Autodesk Inventor part; units mm, degrees
ref_plane "Plano de trabalho1" through (-46, 6, -51.528) normal (0, -1, 0) x (1, 0, 0)
ref_plane "YZ Plane" through (0, 0, 0) normal (1, 0, 0) x (0, 1, 0)
ref_plane "XZ Plane" through (0, 0, 0) normal (0, 1, 0) x (-1, 0, 0)
ref_plane "Plano de trabalho1" through (-46, 6, -51.528) normal (0, -1, 0) x (1, 0, 0)
sketch "Esboço5" plane through (0, 0, 0) normal (0, 1, 0) x (-1, 0, 0)
  line L0 (51.75, 50.222) -> (51.75, -56.778)
  line L1 (38.75, -49.9946) -> (38.75, -21.778)
  line L2 (51.75, -21.778) -> (51.75, -56.778)
  line L3 (38.75, -21.778) -> (-37.25, -21.778)
  line L4 (-37.25, -21.778) -> (-37.25, -49.9946)
  line L5 (-37.25, -49.9946) -> (38.75, -49.9946)
  line L6 (51.75, 50.222) -> (-51.75, 50.222)
  line L7 (-51.75, 50.222) -> (-51.75, -56.778)
  line L8 (-51.75, -56.778) -> (51.75, -56.778)
  point P0 (0, 0)
  dimension "d24" = 76
  dimension "d28" = 51.75
  dimension "d30" = 103.5
extrude "Extrusão4" add sketch "Esboço5" against normal blind 3 from surface at 6
sketch "Esboço6" plane through (-51.75, 3, 50.222) normal (0, -1, 0) x (1, 0, 0)
  point P0 (51.75, -50.222)
sketch "Esboço7" plane through (-51.75, 3, 50.222) normal (0, -1, 0) x (1, 0, 0)
  line L0 (99, -95.2) -> (102, -95.2)
  line L1 (102, -83.2) -> (102, -95.2)
  line L2 (102, -83.2) -> (99, -83.2)
  line L3 (99, -83.2) -> (99, -95.2)
  line L4 (99, -71.4) -> (102, -71.4)
  line L5 (102, -59.4) -> (102, -71.4)
  line L6 (102, -59.4) -> (99, -59.4)
  line L7 (99, -59.4) -> (99, -71.4)
  line L8 (102, -35.6) -> (99, -35.6)
  line L9 (99, -35.6) -> (99, -47.6)
  line L10 (99, -47.6) -> (102, -47.6)
  line L11 (102, -35.6) -> (102, -47.6)
  line L12 (102, -11.8) -> (99, -11.8)
  line L13 (99, -11.8) -> (99, -23.8)
  line L14 (99, -23.8) -> (102, -23.8)
  line L15 (102, -11.8) -> (102, -23.8)
  line L16 (102, -95.2) -> (99, -95.2)
  line L17 (99, -95.2) -> (99, -83.2)
  line L18 (99, -83.2) -> (102, -83.2)
  line L19 (102, -83.2) -> (102, -95.2)
  line L20 (102, -71.4) -> (99, -71.4)
  line L21 (99, -71.4) -> (99, -59.4)
  line L22 (99, -59.4) -> (102, -59.4)
  line L23 (102, -59.4) -> (102, -71.4)
  line L24 (102, -47.6) -> (99, -47.6)
  line L25 (99, -47.6) -> (99, -35.6)
  line L26 (99, -35.6) -> (102, -35.6)
  line L27 (102, -35.6) -> (102, -47.6)
  line L28 (102, -23.8) -> (99, -23.8)
  line L29 (99, -23.8) -> (99, -11.8)
  line L30 (99, -11.8) -> (102, -11.8)
  line L31 (102, -11.8) -> (102, -23.8)
  point P0 (51.75, -50.222)
extrude "Extrusão5" cut sketch "Esboço7" against normal blind 3
equation "\"d30\" = 2 * d28"
properties part number "Chassi_inf"
Input: part model. Units: mm. Frame: model coordinates. A direction names the side the tool comes from. Give positions to 0.01 mm unless a question says otherwise; leave off trailing zeros. Write each loop counter-clockwise with the first axis right and the second up, starting at its lowest first coordinate (ties: lowest second). Pieces come first, ordered by that corner, then holes. Notation, with made-up numbers: (73, 73.25) - (99, 73.25) arc R6 ccw to (99, 81.25) - close; hole circle Ø9 at (18, 27). An arc over 180 degrees is marked (long way). Write item = value, one per line. Start each with the question number.
1. Section query B-B, the plane y = 5.25. Output: boundary loops of the cut face in (x, z), then the cut area to 3 significant figures.
2. Section query A-A, the plane x = -18.5. Output: boundary loops of the cut face in (y, z), then the cut area to 3 significant figures.
3. Section query C-C, the plane z = -24. Output: boundary loops of the cut face in (x, y), then the cut area to 3 significant figures.
4. Access query for faces 4 (the flat face through (50.25, 4, -15)), 5 (the flat face through (-51.75, 5, -3)). Directions: +Z, -Z, +X, -X, +Y, -Y. A direction counts if a zero-diameter tool reaches every point of the face in a straight line with its end or side. Return the directions, or none.
5. First-contact query: pin 1 Ø2 at (x, z) = (20.5, -23.5) entering from +Y. Flat tip, straight axial feed; report the tip coordinate or a pass-through.
6. Mould query, pull axis Z, two halves, no side actions, for faces 1 (the flat face through (50.25, 4, -39)), 2 (the flat face through (1, 6, 9)), 3 (the flat face through (-1, 5, 50.222)). Classes: released by +Z, released by -Z, zero draft, split by the parting line, or undercut.
7. Ray query, L1, parallel to X at y = 4.05, z = -42; L2, parallel to X at y = 3.3, z = 10.5; L3, parallel to Z at x = 23, y = 3.8. Return the intervals inside material, ascending.
Check sheet entries:
q1.outline = (-51.75, -56.78) - (51.75, -56.78) - (51.75, 50.22) - (-51.75, 50.22) - close; hole (-38.75, -49.99) - (37.25, -49.99) - (37.25, -21.78) - (-38.75, -21.78) - close; hole (47.25, -44.98) - (50.25, -44.98) - (50.25, -32.98) - (47.25, -32.98) - close; hole (47.25, -21.18) - (50.25, -21.18) - (50.25, -9.18) - (47.25, -9.18) - close; hole (47.25, 2.62) - (50.25, 2.62) - (50.25, 14.62) - (47.25, 14.62) - close; hole (47.25, 26.42) - (50.25, 26.42) - (50.25, 38.42) - (47.25, 38.42) - close
q1.area = 8,790 mm2
q2.outline = (3, -56.78) - (6, -56.78) - (6, -49.99) - (3, -49.99) - close; (3, -21.78) - (6, -21.78) - (6, 50.22) - (3, 50.22) - close
q2.area = 236 mm2
q3.outline = (-51.75, 3) - (-38.75, 3) - (-38.75, 6) - (-51.75, 6) - close; (37.25, 3) - (51.75, 3) - (51.75, 6) - (37.25, 6) - close
q3.area = 82.5 mm2
q4.face_4 = +Y, -Y
q4.face_5 = +Z, -Z, -X, +Y, -Y
q5.pin_1 = through
q6.face_1 = undercut
q6.face_2 = zero draft
q6.face_3 = released by +Z
q7.L1 = -51.75 to -38.75, 37.25 to 47.25, 50.25 to 51.75
q7.L2 = -51.75 to 47.25, 50.25 to 51.75
q7.L3 = -56.78 to -49.99, -21.78 to 50.22
